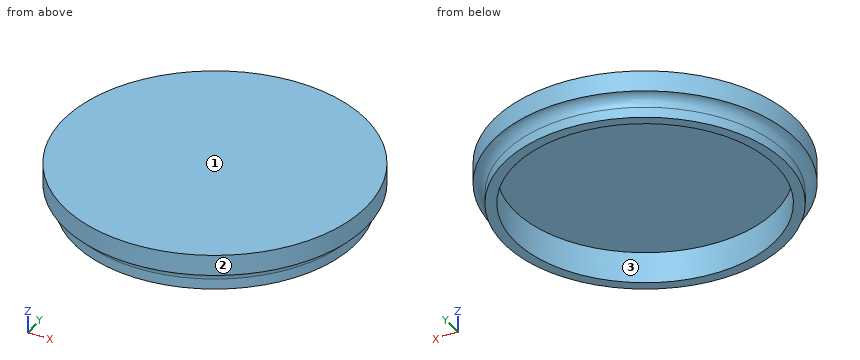
```python
from build123d import *

# Parameters (mm, degrees)
F0_W   = 25
F0_H   = 2
F0_W_2 = 2
F0_H_2 = 4
F2_R   = 1.99999


# Not quite as in the source:
# - a fillet or chamfer is up to 0.001 mm smaller than in the source, because OpenCascade refuses the exact size


with BuildPart() as f1:
    # F0 (on Right) → F1 (revolve)
    with BuildSketch(Plane.YZ):
        with Locations((-12.5, -1)):
            Rectangle(F0_W, F0_H)
        Polygon((-27, -4), (-25, -4), (-25, -2), (-25, 0), (-29, 0), (-29, -4), align=None)
        with Locations((-26, -6)):
            Rectangle(F0_W_2, F0_H_2)
    revolve(axis=Axis((0, 0, -1), (0, 0, -1)))

    # F2 (radius 2 in the source; OpenCascade refuses exactly that, so slightly less here)
    f2_edges = [f1.edges().sort_by_distance(p)[0] for p in [
        (0, 27, -4),
    ]]
    fillet(f2_edges, radius=F2_R)


solid = f1.part
```
Verification items for the finished model (mm, model axes). Face numbers are marked on the shaded views. Round coordinates to 2 decimals unless told otherwise and drop trailing zeros. Write each loop counter-clockwise with the first axis right and the second up, starting at its lowest first coordinate (ties: lowest second). Pieces come first, ordered by that corner, then holes. Notation, with made-up numbers: (49.25, -26) -> (91.25, -26) arc R23 ccw to (91.25, -17) -> close; hole circle Ø2 at (66.25, 85.5). An arc over 180 degrees is marked (long way). Write each question's results on one line, items separated by ' | '. Start each with the question number.
1. Material ranges on probe 1 along Y at (x, z) = (0, -6.25); probe 2 along Z at (x, y) = (13.5, -2), recorded low to high. Write a range as from..to.
2. Depth check by flat-ended pin: P1, Ø3, axis at y = -22, z = -7, coming from the -X side; P2, Ø25, axis at x = 8.5, y = 5, coming from the -Z side; P3, Ø1, axis at y = -1, z = -3.5, coming from the -X side. Enter the tip coordinate at first touch or a pass-through.
3. Draft check along X on the marked faces 1, 2 and 3. Enter one of: +X half, -X half, draft (parallel to the pull), parting line (faces both ways), or undercut.
4. Cross-section at C-C (z = -1). Enter the section's corners in (x, y), then the cut area to 3 significant figures.
Solutions:
1) probe 1: y = -27..-25, 25..27 | probe 2: z = -2..0
2) P1: stops at x = -17.57 | P2: stops at z = -2 | P3: stops at x = -29
3) face 1: draft | face 2: parting line | face 3: undercut
4) outline: circle Ø58 at (0, 0) | area: 2,640 mm2
